Could you check a few things on this model? Use its own coordinates, in mm. A direction names the side the tool comes from. Coordinates: 2 decimals unless noted, no trailing zeros. Order: outer loops, then holes, each group sorted by start corner. A loop starts at its lowest first (then second) coordinate and runs counter-clockwise, first axis right, second up. Notation, with made-up numbers: (20, 48) -> (65, 48) arc R19 ccw to (65, 55) -> close; hole circle Ø9 at (68.25, 44.25). An arc over 180 degrees is marked (long way). Use a Markdown table: item, result. Add a question column.
1) Which directions (+Z, -Z, +X, -X, +Y, -Y) give clear straight access to the entire face, cutting with the end or side of a thin tool? Please do faces 1 (the flat face through (2, 0, -39)), 2 (the flat face through (2, -2, -61)), 3 (the flat face through (2, 9, 0)).
2) If I drill on L1, parallel to Y at x = 3.2, z = -43; L2, parallel to Y at x = 2.45, z = -62; L3, parallel to Z at x = 1.1, y = 37, over which ranges is the centre line in solid material (lowest first)? Write a range as [from, to].
3) Thinking about a two-plate mould opening in Z: for faces 4 (the flat face through (2, -2, -16)), 5 (the flat face through (2, -2, -31)), 6 (the flat face through (0, 15, -25)), 7 (the flat face through (1.97, 21.8, -34.51)), which applies, +Z half, -Z half, draft (parallel to the pull), parting line (faces both ways), or undercut?
4) If we section it at C-C (y = 24): Write out the boundary of the cut face in (x, z), plus the area to 3 significant figures.
5) If we section it at B-B (z = -24.5): Write out the boundary of the cut face in (x, y).
6) If we section it at A-A (x = 2.15): Write out the boundary of the cut face in (y, z), plus the area to 4 significant figures.
7) Will these pins go through, and if not, where does the flat tip stop? pin 1 Ø2 at (x, y) = (1, -2) entering from -Z; pin 2 Ø2 at (x, z) = (3, -7.5) entering from -Y; pin 3 Ø1.2 at (x, y) = (3, 10) entering from +Z.
```python
from build123d import *

# Parameters (mm, degrees)
SKETCH1_W           = 15
SKETCH1_H           = 4
SKETCH1_W_2         = 4
SKETCH1_H_2         = 25
BOSS_EXTRUDE1_DEPTH = 4


with BuildPart() as part:
    # Sketch1 → Boss-Extrude1 (new body)
    with BuildSketch(Plane(origin=(0, 0, 0), x_dir=(0, 0, -1), z_dir=(1, 0, 0))):
        Polygon((70, 0), (0, 0), (0, 43), align=None)
        with Locations((53.5, -2)):
            Rectangle(SKETCH1_W, SKETCH1_H)
        with Locations((23.5, -2)):
            Rectangle(SKETCH1_W, SKETCH1_H)
        with Locations((-2, 30.5)):
            Rectangle(SKETCH1_W_2, SKETCH1_H_2)
    extrude(amount=BOSS_EXTRUDE1_DEPTH)


solid = part.part
```
Answer sheet:
| question | item | result |
|---|---|---|
| 1 | face 1 | +X, -X, -Y |
| 1 | face 2 | -Z, +X, -X, -Y |
| 1 | face 3 | +Z, +X, -X, -Y |
| 2 | L1 | [0, 16.59] |
| 2 | L2 | [0, 4.91] |
| 2 | L3 | [-9.77, 4] |
| 3 | face 4 | +Z half |
| 3 | face 5 | undercut |
| 3 | face 6 | draft |
| 3 | face 7 | -Z half |
| 4 | outline | (0, -30.93) -> (4, -30.93) -> (4, 4) -> (0, 4) -> close |
| 4 | area | 140 mm2 |
| 5 | outline | (0, -4) -> (4, -4) -> (4, 27.95) -> (0, 27.95) -> close |
| 6 | outline | (-4, -61) -> (0, -61) -> (0, -70) -> (43, 0) -> (43, 4) -> (18, 4) -> (18, 0) -> (0, 0) -> (0, -16) -> (-4, -16) -> (-4, -31) -> (0, -31) -> (0, -46) -> (-4, -46) -> close |
| 6 | area | 1,725 mm2 |
| 7 | pin 1 | z = -61 |
| 7 | pin 2 | y = 0 |
| 7 | pin 3 | z = 0 |
